Design review of the part shown in the three views and the two pictorial views. Dimensions are in mm from the part's minimum x, y and z. Coordinates: 2 decimals unless noted, no trailing zeros. Write each loop counter-clockwise with the first axis right and the second up, starting at its lowest first coordinate (ties: lowest second). Pieces come first, ordered by that corner, then holes.
Q1. Take a section at A-A, the plane x = 45. Write out the cut boundary in (y, z).
Q2. Take a section at D-D, the plane x = 6.5. Write out the cut boundary in (y, z), plus the area to 3 significant figures.
Q3. For L1, parallel to Y at x = 6.5, z = 1.55; L2, parallel to X at y = 61, z = 2.9; L3, parallel to Y at x = 45, z = 1.9, list the stretches that pass through material, from the lowest coordinate up.
Q4. Take a section at C-C, the plane z = 0.7. Write out the cut boundary in (x, y).
Q5. For pin 1 Ø4 at (x, y) = (33.5, 6.5) entering from +Z; pin 2 Ø0.9 at (x, z) = (67.5, 1.5) entering from -Y; pin 3 Ø1.5 at (y, z) = (29, 2.5) entering from +X, all flat-tipped, find the tip position at first contact; note any pin that passes through.
Q6. Take a section at B-B, the plane y = 6.5. Write out the cut boundary in (x, z).
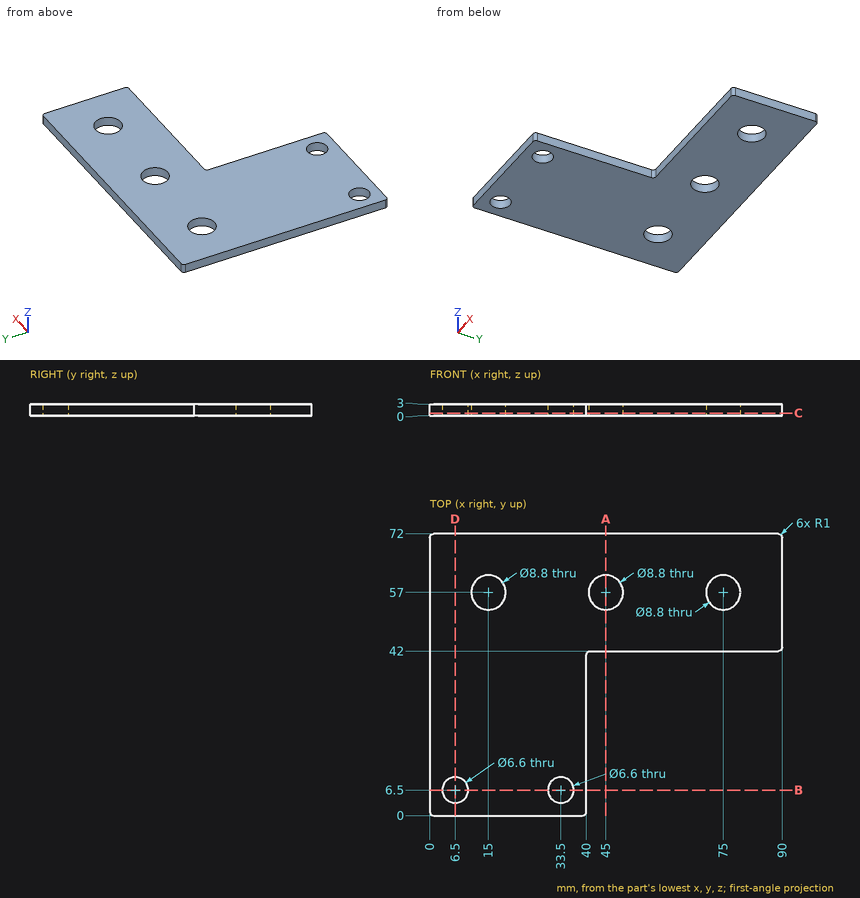
Responses:
1. outline: (42, 0) - (52.6, 0) - (52.6, 3) - (42, 3) - close; (61.4, 0) - (72, 0) - (72, 3) - (61.4, 3) - close
2. outline: (0, 0) - (3.2, 0) - (3.2, 3) - (0, 3) - close; (9.8, 0) - (72, 0) - (72, 3) - (9.8, 3) - close
2. area: 196 mm2
3. L1: y = 0 to 3.2, 9.8 to 72
3. L2: x = 0 to 13.17, 16.83 to 43.17, 46.83 to 73.17, 76.83 to 90
3. L3: y = 42 to 52.6, 61.4 to 72
4. outline: (0, 1) arc R1 ccw to (1, 0) - (39, 0) arc R1 ccw to (40, 1) - (40, 41) arc R1 cw to (41, 42) - (89, 42) arc R1 ccw to (90, 43) - (90, 71) arc R1 ccw to (89, 72) - (1, 72) arc R1 ccw to (0, 71) - close; hole circle Ø6.6 at (6.5, 6.5); hole circle Ø8.8 at (15, 57); hole circle Ø6.6 at (33.5, 6.5); hole circle Ø8.8 at (45, 57); hole circle Ø8.8 at (75, 57)
5. pin 1: passes through
5. pin 2: stops at y = 42
5. pin 3: stops at x = 40
6. outline: (0, 0) - (3.2, 0) - (3.2, 3) - (0, 3) - close; (9.8, 0) - (30.2, 0) - (30.2, 3) - (9.8, 3) - close; (36.8, 0) - (40, 0) - (40, 3) - (36.8, 3) - close
